For this review, take the finished solid that the model builds, in its own axes (mm). A direction names the side the tool comes from. Give positions to 0.01 mm unless a question says otherwise; leave off trailing zeros. Order: outer loops, then holes, each group sorted by start corner. A loop starts at its lowest first (then second) coordinate and runs counter-clockwise, first axis right, second up.
Item 1: Machinability: for faces 4 (the flat face through (55, 0, 11)), 5 (the flat face through (-34.5, 64, 11)), 6 (the flat face through (47.028, 81.455, 9.916)), 7 (the flat face through (-64.9, 68.1, 4.25)), which of the approach directions +Z, -Z, +X, -X, +Y, -Y give a long, thin tool a straight path to every point of the face, cutting with its end or side? Answer none if there is none.
Item 2: Consider section D-D (y = 45). Give the boundary of the cut face in (x, z).
Item 3: Consider section A-A (z = 8.5). Give the number of separate pieces and of enclosed holes in the cut face, plus the area to 3 significant figures.
Item 4: Consider section C-C (y = -56). Give the boundary of the cut face in (x, z), plus the area to 3 significant figures.
Item 5: The part is to be moulded in two halves that separate along X. For faces 1 (the cylindrical face through (-42.29, 36.03, 11.4)), 2 (the flat face through (15, -89, 16)), 3 (the flat face through (-47.028, 81.455, 9.916)), say which applies: released by +X, released by -X, zero draft, split by the parting line, or undercut.
Item 6: For probe 1 along Y at (x, z) = (0, 8); probe 2 along X at (y, z) = (34, 17.9); probe 3 along Y at (x, z) = (4.5, 16.9), list the stretches that pass through material, from the lowest coordinate up.
Item 7: For P1, Ø4, axis at x = 71.5, z = 15, coming from the -Y side; P2, Ø5, axis at x = 66.468, y = 66.468, coming from the +Z side; P3, Ø5, axis at x = -45.5, z = 13, coming from the +Y side, all flat-tipped, find the tip position at first contact; note any pin that passes through.
Item 8: Consider section B-B (y = 0). Give the boundary of the cut face in (x, z), plus the area to 3 significant figures.
Autodesk Fusion 360 part; units mm, degrees
sketch "Sketch1" plane through (0, 0, 0) normal (0, 0, 1) x (1, 0, 0)
  circle A0 centre (0, 0) radius 102
  dimension "d1" = 204
extrude "Extrude1" add sketch "Sketch1" along normal blind 4
sketch "Sketch2" plane through (0, 0, 4) normal (0, 0, 1) x (-1, 0, 0)
  circle A0 centre (0, 0) radius 102
  line L0 (0, 0) -> (0, -98) construction
  circle A1 centre (0, 0) radius 94 construction
  line L1 (0, 0) -> (-49, -84.8705) construction
  line L2 (0, 0) -> (98, 0) construction
  line L3 (0, 0) -> (-62.9932, -75.0724) construction
  line L4 (0, 0) -> (98, 0) construction
  line L5 (0, 0) -> (49, -84.8705) construction
  line L6 (0, 0) -> (98, 0) construction
  line L7 (0, 0) -> (62.9932, -75.0724) construction
  line L8 (0, 0) -> (98, 0) construction
  line L9 (62.9932, -75.0724) -> (57.8509, -68.944)
  line L10 (49, -84.8705) -> (45, -77.9423)
  line L11 (-49, -84.8705) -> (-45, -77.9423)
  line L12 (-62.9932, -75.0724) -> (-57.8509, -68.944)
  arc A2 (62.9932, -75.0724) -> (-62.9932, -75.0724) centre (0, 0) ccw
  arc A3 (-49, -84.8705) -> (49, -84.8705) centre (0, 0) ccw
  arc A4 (57.8509, -68.944) -> (-57.8509, -68.944) centre (0, 0) ccw
  arc A5 (-45, -77.9423) -> (45, -77.9423) centre (0, 0) ccw
  line L13 (0, 0) -> (0, -64) construction
  line L14 (34.5, -79) -> (-34.5, -79)
  line L15 (-34.5, -79) -> (-34.5, -49)
  line L16 (-34.5, -49) -> (34.5, -49)
  line L17 (34.5, -49) -> (34.5, -79)
  line L18 (34.5, -79) -> (-34.5, -49) construction
  line L19 (-34.5, -79) -> (34.5, -49) construction
  line L20 (36, -80) -> (-36, -80)
  line L21 (-36, -80) -> (-36, -48)
  line L22 (-36, -48) -> (36, -48)
  line L23 (36, -48) -> (36, -80)
  line L24 (36, -80) -> (-36, -48) construction
  line L25 (-36, -80) -> (36, -48) construction
  line L26 (0, 0) -> (-63, 0) construction
  line L27 (-55, -19) -> (-71, -19)
  line L28 (-71, -19) -> (-71, 19)
  line L29 (-71, 19) -> (-55, 19)
  line L30 (-55, 19) -> (-55, -19)
  line L31 (-55, -19) -> (-71, 19) construction
  line L32 (-71, -19) -> (-55, 19) construction
  line L33 (0, 0) -> (0, 5) construction
  line L34 (0, 5) -> (20, 5) construction
  line L35 (48, -37.5) -> (-8, -37.5) construction
  line L36 (-8, -37.5) -> (-8, 47.5) construction
  line L37 (-8, 47.5) -> (48, 47.5) construction
  line L38 (48, 47.5) -> (48, -37.5) construction
  line L39 (48, -37.5) -> (-8, 47.5) construction
  line L40 (-8, -37.5) -> (48, 47.5) construction
  line L41 (0, 0) -> (48, -37.5) construction
  line L42 (0, 0) -> (48, 47.5) construction
  line L43 (0, 0) -> (49, 0) construction
  line L44 (0, 0) -> (0, 47.5) construction
  line L45 (0, 0) -> (-8, 47.5) construction
  line L46 (0, 0) -> (-8, 0) construction
  line L47 (0, 0) -> (-8, -37.5) construction
  line L48 (0, 0) -> (-71, -19) construction
  line L49 (0, 0) -> (-71, 19) construction
  circle A6 centre (0, -94) radius 2
  circle A7 centre (0, 94) radius 2
  line L50 (0, 0) -> (66.468, -66.468) construction
  line L51 (0, 0) -> (94, 0) construction
  line L52 (0, 0) -> (-66.468, -66.468) construction
  line L53 (0, 0) -> (94, 0) construction
  circle A8 centre (66.468, -66.468) radius 2 construction
  circle A9 centre (-66.468, -66.468) radius 2 construction
  line L54 (0, 0) -> (-66.468, 66.468) construction
  line L55 (0, 0) -> (94, 0) construction
  circle A10 centre (-66.468, 66.468) radius 2 construction
  line L56 (0, 0) -> (66.468, 66.468) construction
  line L57 (0, 0) -> (94, 0) construction
  circle A11 centre (66.468, 66.468) radius 2 construction
  line L58 (0, 0) -> (24.329, -90.797) construction
  line L59 (0, 0) -> (94, 0) construction
  line L60 (0, 0) -> (-47, 81.4064) construction
  line L61 (0, 0) -> (94, 0) construction
  circle A12 centre (66.468, -66.468) radius 2
  circle A13 centre (-66.468, -66.468) radius 2
  circle A14 centre (66.468, 66.468) radius 2
  circle A15 centre (-66.468, 66.468) radius 2
  point P0 (0, -64)
  point P1 (0, -64)
  point P2 (-63, 0)
  point P3 (20, 5)
  dimension "d4" = 180
  dimension "d5" = 196
  dimension "d6" = 188
  dimension "d7" = 120
  dimension "d8" = 130
  dimension "d9" = 60
  dimension "d10" = 50
  dimension "d11" = 64
  dimension "d12" = 69
  dimension "d13" = 30
  dimension "d14" = 72
  dimension "d15" = 32
  dimension "d16" = 63
  dimension "d17" = 16
  dimension "d18" = 38
  dimension "d19" = 56
  dimension "d20" = 85
  dimension "d21" = 20
  dimension "d22" = 5
  dimension "d23" = 37.999
  dimension "d24" = 44.7
  dimension "d25" = 45.3
  dimension "d26" = 9.56
  dimension "d27" = 14.982
  dimension "d28" = 14.982
  dimension "d29" = 4
  dimension "d30" = 4
  dimension "d31" = 45
  dimension "d32" = 135
  dimension "d33" = 4
  dimension "d34" = 4
  dimension "d35" = 135
  dimension "d36" = 94
  dimension "d37" = 4
  dimension "d38" = 45
  dimension "d39" = 4
  dimension "d40" = 75
  dimension "d41" = 120
  dimension "d42" = 4
  dimension "d43" = 4
  dimension "d44" = 4
  dimension "d45" = 4
extrude "Extrude2" add sketch "Sketch2" along normal blind 12 contours L9 L12 A2 A4 | L10 L11 A3 A5
sketch "Sketch3" plane through (0, 0, 0) normal (0, 0, -1) x (1, 0, 0)
  circle A0 centre (0, 0) radius 102
  circle A1 centre (0, 0) radius 94 construction
  line L0 (0, 0) -> (-66.468, -66.468) construction
  line L1 (0, 0) -> (94, 0) construction
  line L2 (0, 0) -> (0, -94) construction
  line L3 (0, 0) -> (66.468, -66.468) construction
  line L4 (0, 0) -> (94, 0) construction
  line L5 (0, 0) -> (0, -94) construction
  line L6 (0, 0) -> (66.468, 66.468) construction
  line L7 (0, 0) -> (94, 0) construction
  line L8 (0, 0) -> (0, 94) construction
  line L9 (0, 0) -> (-66.468, 66.468) construction
  line L10 (0, 0) -> (94, 0) construction
  line L11 (150, 0) -> (-200, 0) construction
  circle A2 centre (0, -94) radius 3.75
  circle A3 centre (66.468, -66.468) radius 3.75
  circle A4 centre (-66.468, -66.468) radius 3.75
  circle A5 centre (66.468, 66.468) radius 3.75
  circle A6 centre (0, 94) radius 3.75
  circle A7 centre (-66.468, 66.468) radius 3.75
  dimension "d48" = 188
  dimension "d49" = 135
  dimension "d50" = 45
  dimension "d51" = 45
  dimension "d52" = 135
  dimension "d53" = 7.5
  dimension "d54" = 7.5
  dimension "d55" = 7.5
extrude "Extrude3" cut sketch "Sketch3" against normal blind 4.25 contours A2 | A3 | A4 | A5 | A6 | A7
extrude "Extrude4" add sketch "Sketch2" along normal blind 14 contours L20 L21 L22 L23 | L27 L28 L29 L30
sketch "Sketch4" plane through (0, 0, 4) normal (0, 0, 1) x (-1, 0, 0)
  line L0 (-49, -84.8705) -> (-45, -77.9423)
  arc A0 (-45, -77.9423) -> (45, -77.9423) centre (0, 0) ccw
  line L1 (45, -77.9423) -> (49, -84.8705)
  arc A1 (-49, -84.8705) -> (49, -84.8705) centre (0, 0) ccw
  circle A2 centre (0, 0) radius 102
  line L2 (62.9932, -75.0724) -> (57.8509, -68.944)
  arc A3 (57.8509, -68.944) -> (-57.8509, -68.944) centre (0, 0) ccw
  line L3 (-57.8509, -68.944) -> (-62.9932, -75.0724)
  arc A4 (62.9932, -75.0724) -> (-62.9932, -75.0724) centre (0, 0) ccw
  line L4 (-55, 19) -> (-55, -19)
  line L5 (-55, -19) -> (-71, -19)
  line L6 (-71, -19) -> (-71, 19)
  line L7 (-71, 19) -> (-55, 19)
  line L8 (36, -48) -> (36, -80)
  line L9 (36, -80) -> (-36, -80)
  line L10 (-36, -80) -> (-36, -48)
  line L11 (-36, -48) -> (36, -48)
  line L12 (0, 0) -> (0, 5) construction
  line L13 (0, 5) -> (20, 5) construction
  line L14 (48, -37.5) -> (-8, -37.5) construction
  line L15 (-8, -37.5) -> (-8, 47.5) construction
  line L16 (-8, 47.5) -> (48, 47.5) construction
  line L17 (48, 47.5) -> (48, -37.5) construction
  line L18 (48, -37.5) -> (-8, 47.5) construction
  line L19 (-8, -37.5) -> (48, 47.5) construction
  line L20 (20, 47.5) -> (20, -37.5) construction
  line L21 (48, 5) -> (0, 5) construction
  line L22 (48, -37.5) -> (44.5, -37.5) construction
  line L23 (44.5, -37.5) -> (44.5, -34) construction
  line L24 (44.5, -34) -> (44.5, 24) construction
  circle A5 centre (44.5, -34) radius 3
  circle A6 centre (44.5, 24) radius 3
  circle A7 centre (-4.5, -34) radius 3
  circle A8 centre (-4.5, 24) radius 3
  line L25 (-4.5, -34) -> (-4.5, -5) construction
  line L26 (-2, -30) -> (-7, -30) construction
  line L27 (-7, -30) -> (-7, 20) construction
  line L28 (-7, 20) -> (-2, 20) construction
  line L29 (-2, 20) -> (-2, -30) construction
  line L30 (-2, -30) -> (-7, 20) construction
  line L31 (-7, -30) -> (-2, 20) construction
  line L32 (0, 0) -> (0, -5) construction
  line L33 (0, -5) -> (-4.5, -5) construction
  point P0 (20, 5)
  point P1 (-4.5, -5)
  dimension "d60" = 5
  dimension "d61" = 20
  dimension "d62" = 56
  dimension "d63" = 85
  dimension "d64" = 3.5
  dimension "d65" = 3.5
  dimension "d66" = 58
  dimension "d67" = 6
  dimension "d68" = 6
  dimension "d69" = 29
  dimension "d70" = 5
  dimension "d71" = 50
  dimension "d72" = 5
  dimension "d73" = 4.5
extrude "Extrude5" add sketch "Sketch4" along normal blind 15 contours A5 | A6 | A7 | A8
sketch "Sketch5" plane through (0, 0, 19) normal (0, 0, 1) x (-1, 0, 0)
  circle A0 centre (44.5, 24) radius 3
  circle A1 centre (44.5, 24) radius 1.6
  dimension "d76" = 3.2
sketch "Sketch6" plane through (0, 0, 19) normal (0, 0, 1) x (-1, 0, 0)
  circle A0 centre (44.5, -34) radius 3
  circle A1 centre (44.5, -34) radius 1.6
  dimension "d77" = 3.2
sketch "Sketch7" plane through (0, 0, 19) normal (0, 0, 1) x (-1, 0, 0)
  circle A0 centre (-4.5, -34) radius 3
  circle A1 centre (-4.5, -34) radius 1.6
  dimension "d78" = 3.2
sketch "Sketch8" plane through (0, 0, 19) normal (0, 0, 1) x (-1, 0, 0)
  circle A0 centre (-4.5, 24) radius 3
  circle A1 centre (-4.5, 24) radius 1.6
  dimension "d79" = 3.2
extrude "Extrude6" cut sketch "Sketch5" sketch "Sketch7" sketch "Sketch6" sketch "Sketch8" against normal blind 5 contours A1 of sketch 2 contours A1 of sketch 3 contours A1 of sketch 4 contours A1
sketch "Sketch9" plane through (0, 0, 16) normal (0, 0, 1) x (-1, 0, 0)
  circle A0 centre (66.468, -66.468) radius 2
  circle A1 centre (-66.468, 66.468) radius 2
  circle A2 centre (-66.468, -66.468) radius 2
  circle A3 centre (66.468, 66.468) radius 2
  circle A4 centre (0, 94) radius 2
  arc A5 (62.9932, -75.0724) -> (-62.9932, -75.0724) centre (0, 0) ccw
  line L0 (-62.9932, -75.0724) -> (-57.8509, -68.944)
  arc A6 (57.8509, -68.944) -> (-57.8509, -68.944) centre (0, 0) ccw
  line L1 (57.8509, -68.944) -> (62.9932, -75.0724)
  line L2 (0, 0) -> (94, 0) construction
  line L3 (0, 0) -> (94, 0) construction
Resolved:
1. face 4: +Z, +Y
1. face 5: +Z
1. face 6: +Z, +X
1. face 7: -Z
2. outline: (-91.54, 0) - (91.54, 0) - (91.54, 4) - (87.06, 4) - (87.06, 16) - (77.94, 16) - (77.94, 4) - (-77.94, 4) - (-77.94, 16) - (-87.06, 16) - (-87.06, 4) - (-91.54, 4) - close
3. separate pieces: 8
3. enclosed holes: 7
3. area: 5,340 mm2
4. outline: (-85.25, 0) - (85.25, 0) - (85.25, 4) - (80.42, 4) - (80.42, 16) - (70.46, 16) - (70.46, 4) - (-70.46, 4) - (-70.46, 16) - (-80.42, 16) - (-80.42, 4) - (-85.25, 4) - close
4. area: 921 mm2
5. face 1: undercut
5. face 2: zero draft
5. face 3: released by -X
6. probe 1: y = -98 to -96, -92 to -90, 48 to 49, 79 to 80, 90 to 92, 96 to 98
6. probe 2: x = -47.5 to -46.1, -42.9 to -41.5, 1.5 to 2.9, 6.1 to 7.5
6. probe 3: y = -27 to -25.6, -22.4 to -21, 31 to 32.4, 35.6 to 37, 48 to 49, 79 to 80
7. P1: stops at y = -69.09
7. P2: stops at z = 16
7. P3: stops at y = 88.06
8. outline: (-102, 0) - (102, 0) - (102, 4) - (98, 4) - (98, 16) - (90, 16) - (90, 4) - (71, 4) - (71, 18) - (55, 18) - (55, 4) - (-90, 4) - (-90, 16) - (-98, 16) - (-98, 4) - (-102, 4) - close
8. area: 1,230 mm2
